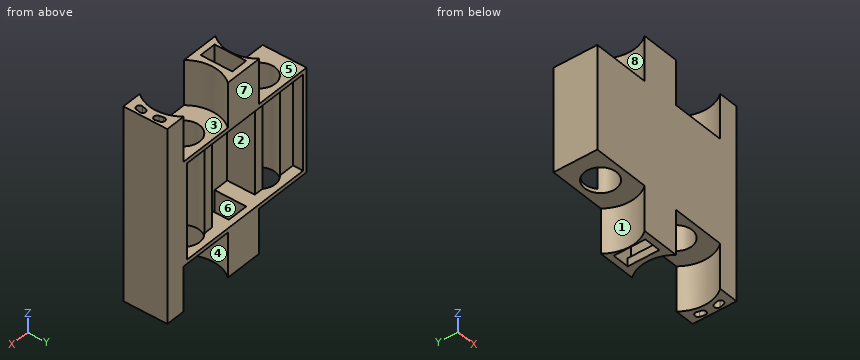
from build123d import *

# Parameters (mm, degrees)
SKETCH1_W           = 95
SKETCH1_H           = 95
BOSS_EXTRUDE1_DEPTH = 25
SKETCH2_R           = 7.75
CUT_EXTRUDE2_DEPTH  = 100
SKETCH3_R           = 17
CUT_EXTRUDE3_DEPTH  = 22
CUT_EXTRUDE4_START  = -22
SKETCH4_R           = 17
CUT_EXTRUDE4_DEPTH  = 22
SKETCH5_W           = 6.246993927
SKETCH5_H           = 25
CUT_EXTRUDE5_DEPTH  = 22
SKETCH6_W           = 7.178723585
SKETCH6_H           = 25
CUT_EXTRUDE6_DEPTH  = 22
SKETCH8_W           = 99.503929421
SKETCH8_H           = 3.5
CUT_EXTRUDE7_DEPTH  = 100
SKETCH9_W           = 8.3
SKETCH9_H           = 15.5
CUT_EXTRUDE11_DEPTH = 100
SKETCH13_W          = 87
SKETCH13_H          = 15.5
CUT_EXTRUDE12_DEPTH = 2
SKETCH14_W          = 25.5
SKETCH14_H          = 47
CUT_EXTRUDE14_DEPTH = 18.5
SKETCH16_W          = 24.75
SKETCH16_H          = 47
CUT_EXTRUDE15_DEPTH = 5
SKETCH17_W          = 20.919567191
SKETCH17_H          = 47
CUT_EXTRUDE16_DEPTH = 5
CUT_EXTRUDE17_DEPTH = 100
FILLET6_R           = 1.5
FILLET7_R           = 1.5
FILLET8_R           = 1.5
FILLET9_R           = 1.5
SKETCH19_W          = 12.12120401
SKETCH19_H          = 21.5
CUT_EXTRUDE20_DEPTH = 100


with BuildPart() as part:
    # Sketch1 → Boss-Extrude1 (new body)
    with BuildSketch(Plane(origin=(0, 0, 0), x_dir=(1, 0, 0), z_dir=(0, 1, 0))):
        with Locations((3.271948822, -17.506298191)):
            Rectangle(SKETCH1_W, SKETCH1_H)
    extrude(amount=BOSS_EXTRUDE1_DEPTH)

    # Sketch2 → Cut-Extrude2 (cut)
    with BuildSketch(Plane.XY.offset(65.006298191)):
        with Locations((-29.228051178, 10.75)):
            Circle(SKETCH2_R)
        with Locations((15.771948822, 10.75)):
            Circle(SKETCH2_R)
    extrude(amount=-CUT_EXTRUDE2_DEPTH, mode=Mode.SUBTRACT)

    # Sketch3 → Cut-Extrude3 (cut)
    with BuildSketch(Plane.XY.offset(65.006298191)):
        with Locations((-29.228051178, 10.75)):
            Circle(SKETCH3_R)
        with Locations((15.771948822, 10.75)):
            Circle(SKETCH3_R)
    extrude(amount=-CUT_EXTRUDE3_DEPTH, mode=Mode.SUBTRACT)

    # Sketch4 → Cut-Extrude4 (cut)
    with BuildSketch(Plane(origin=(0, 0, -29.993701809), x_dir=(-1, 0, 0), z_dir=(0, 0, -1)).offset(CUT_EXTRUDE4_START)):
        with Locations((-15.771948822, 10.75)):
            Circle(SKETCH4_R)
        with Locations((29.228051178, 10.75)):
            Circle(SKETCH4_R)
    extrude(amount=CUT_EXTRUDE4_DEPTH, mode=Mode.SUBTRACT)

    # Sketch5 → Cut-Extrude5 (cut)
    with BuildSketch(Plane.XY.offset(65.006298191)):
        with Locations((-41.104554214, 12.5)):
            Rectangle(SKETCH5_W, SKETCH5_H)
    extrude(amount=-CUT_EXTRUDE5_DEPTH, mode=Mode.SUBTRACT)

    # Sketch6 → Cut-Extrude6 (cut)
    with BuildSketch(Plane(origin=(0, 0, -29.993701809), x_dir=(-1, 0, 0), z_dir=(0, 0, -1))):
        with Locations((40.638689386, 12.5)):
            Rectangle(SKETCH6_W, SKETCH6_H)
    extrude(amount=-CUT_EXTRUDE6_DEPTH, mode=Mode.SUBTRACT)

    # Sketch8 → Cut-Extrude7 (cut)
    with BuildSketch(Plane(origin=(0, 0, -29.993701809), x_dir=(-1, 0, 0), z_dir=(0, 0, -1))):
        with Locations((-1.019984112, 23.25)):
            Rectangle(SKETCH8_W, SKETCH8_H)
    extrude(amount=-CUT_EXTRUDE7_DEPTH, mode=Mode.SUBTRACT)

    # Sketch9 → Cut-Extrude11 (cut)
    with BuildSketch(Plane.XY.offset(65.006298191)):
        with Locations((-7.828051178, 10.75)):
            Rectangle(SKETCH9_W, SKETCH9_H)
    extrude(amount=-CUT_EXTRUDE11_DEPTH, mode=Mode.SUBTRACT)

    # Sketch13 → Cut-Extrude12 (cut)
    with BuildSketch(Plane.ZY.offset(3.678051178)):
        with Locations((17.506298191, 10.75)):
            Rectangle(SKETCH13_W, SKETCH13_H)
    extrude(amount=-CUT_EXTRUDE12_DEPTH, mode=Mode.SUBTRACT)

    # Sketch14 → Cut-Extrude14 (cut)
    with BuildSketch(Plane(origin=(0, 21.5, 0), x_dir=(1, 0, 0), z_dir=(0, 1, 0))):
        with Locations((-6.728051178, -17.506298191)):
            Rectangle(SKETCH14_W, SKETCH14_H)
    extrude(amount=-CUT_EXTRUDE14_DEPTH, mode=Mode.SUBTRACT)

    # Sketch16 → Cut-Extrude15 (cut)
    with BuildSketch(Plane(origin=(0, 21.5, 0), x_dir=(1, 0, 0), z_dir=(0, 1, 0))):
        with Locations((-29.853051178, -17.506298191)):
            Rectangle(SKETCH16_W, SKETCH16_H)
    extrude(amount=-CUT_EXTRUDE15_DEPTH, mode=Mode.SUBTRACT)

    # Sketch17 → Cut-Extrude16 (cut)
    with BuildSketch(Plane(origin=(0, 21.5, 0), x_dir=(1, 0, 0), z_dir=(0, 1, 0))):
        with Locations((16.481732418, -17.506298191)):
            Rectangle(SKETCH17_W, SKETCH17_H)
    extrude(amount=-CUT_EXTRUDE16_DEPTH, mode=Mode.SUBTRACT)

    # Sketch18 → Cut-Extrude17 (cut)
    with BuildSketch(Plane.XY.offset(65.006298191)):
        with BuildLine():
            Line((34.66639245, 12.75), (37.680851122, 12.75))
            ThreePointArc((37.680851122, 12.75), (37.300376381, 15.28065192), (36.628602437, 17.75))
            Line((36.628602437, 17.75), (33.435470555, 17.75))
            ThreePointArc((33.435470555, 17.75), (34.221100776, 15.291893017), (34.66639245, 12.75))
        make_face()
        with BuildLine():
            Line((34.66639245, 8.75), (37.680851122, 8.75))
            ThreePointArc((37.680851122, 8.75), (37.300376381, 6.21934808), (36.628602437, 3.75))
            Line((36.628602437, 3.75), (33.435470555, 3.75))
            ThreePointArc((33.435470555, 3.75), (34.221100776, 6.208106983), (34.66639245, 8.75))
        make_face()
    extrude(amount=-CUT_EXTRUDE17_DEPTH, mode=Mode.SUBTRACT)

    # Fillet6
    fillet6_edges = [part.edges().sort_by_distance(p)[0] for p in [
        (33.435470555, 17.75, 17.506298191),
        (36.628602437, 17.75, 17.506298191),
    ]]
    fillet(fillet6_edges, radius=FILLET6_R - 0.0001)  # a hair under: the kernel refuses the full size

    # Fillet7
    fillet7_edges = [part.edges().sort_by_distance(p)[0] for p in [
        (37.680851122, 12.75, 17.506298191),
        (34.66639245, 12.75, 17.506298191),
    ]]
    fillet(fillet7_edges, radius=FILLET7_R - 0.0001)  # a hair under: the kernel refuses the full size

    # Fillet8
    fillet8_edges = [part.edges().sort_by_distance(p)[0] for p in [
        (33.435470555, 3.75, 17.506298191),
        (36.628602437, 3.75, 17.506298191),
    ]]
    fillet(fillet8_edges, radius=FILLET8_R - 0.0001)  # a hair under: the kernel refuses the full size

    # Fillet9
    fillet9_edges = [part.edges().sort_by_distance(p)[0] for p in [
        (37.680851122, 8.75, 17.506298191),
        (34.66639245, 8.75, 17.506298191),
    ]]
    fillet(fillet9_edges, radius=FILLET9_R - 0.0001)  # a hair under: the kernel refuses the full size

    # Sketch19 → Cut-Extrude20 (cut)
    with BuildSketch(Plane.XY.offset(65.006298191)):
        with Locations((44.711346817, 10.75)):
            Rectangle(SKETCH19_W, SKETCH19_H)
    extrude(amount=-CUT_EXTRUDE20_DEPTH, mode=Mode.SUBTRACT)


solid = part.part
CAD build for the part. Positions are in the model's coordinates, mm. Face numbers are marked on the shaded views. A direction names the side the tool comes from. Round coordinates to 2 decimals unless told otherwise and drop trailing zeros. Write each loop counter-clockwise with the first axis right and the second up, starting at its lowest first coordinate (ties: lowest second). Pieces come first, ordered by that corner, then holes.
(1) 3-axis set-ups, long thin cutter, end or side, ignore diameter. For the marked faces 1, 2, 3, 4 and 5: which of +Z, -Z, +X, -X, +Y, -Y reach the whole face in a straight line?
(2) Drop flat-ended pins along their axis: P1, Ø3, axis at x = 9.5, z = 31, coming from the +Y side; P2, Ø6.5, axis at x = -23, y = 10.5, coming from the +Z side; P3, Ø8, axis at y = 12.5, z = 51, coming from the -X side; P4, Ø9.5, axis at x = -29.23, y = 10.75, coming from the +Z side. Give the stop position or say it passes through.
(3) Mould opens along X. For the marked faces 6, 7 and 8 say: pulls with the +X half, pulls with the -X half, needs draft (parallel to the pull), parting line crosses it, or undercut.
(4) Slice it at A-A, the plane z = -15. Count the separate pieces of the cut face and the enclosed holes in it, and give its area (3 significant figures).
(5) Probe line 1 along X through (y, z) = (11.25, -8.5); line 2 along X through (y, z) = (16.5, -15.5); line 3 along Z through (x, y) = (-19, 11). List the from-to ranges inside material, lowest first.
(6) Slice it at C-C, the plane x = -29.5. Write the cut outline in (y, z), and give its area (3 significant figures).
From the geometry:
1. face 1: -Z, -X
1. face 2: +Y
1. face 3: +Z
1. face 4: -Z
1. face 5: +Z, -X
2. P1: stops at y = 16.5
2. P2: stops at z = 43.01
2. P3: stops at x = -13.23
2. P4: passes through
3. face 6: undercut
3. face 7: needs draft
3. face 8: pulls with the -X half
4. separate pieces: 2
4. enclosed holes: 3
4. area: 255 mm2
5. line 1: x = -12.24 to -11.98, -1.68 to -1.22, 32.76 to 38.65
5. line 2: x = -13.23 to -11.98, -1.68 to -0.23, 31.77 to 34.04, 37.01 to 38.65
5. line 3: z = -7.99 to -5.99, 41.01 to 43.01
6. outline: (0, -7.99) - (3, -7.99) - (3, 43.01) - (0, 43.01) - close; (18.5, -7.99) - (21.5, -7.99) - (21.5, -5.99) - (18.5, -5.99) - close; (18.5, 41.01) - (21.5, 41.01) - (21.5, 43.01) - (18.5, 43.01) - close
6. area: 165 mm2
